Check sheet for the drawn part. Datum: minimum x, y, z corner. Units: mm. A direction names the side the tool comes from. Give positions to 0.01 mm unless a question says otherwise; leave off trailing zeros. Write each loop counter-clockwise with the first axis right and the second up, starting at its lowest first coordinate (ties: lowest second). Pieces come first, ordered by that corner, then holes.
(1) Depth check by flat-ended pin: P1, Ø2, axis at x = 19.5, z = 4, coming from the -Y side; P2, Ø4, axis at x = 82.5, z = 3.5, coming from the -Y side. Enter the tip coordinate at first touch or a pass-through.
(2) Thickness scan on line 1 along Y through (x, z) = (24, 2); line 2 along X through (y, z) = (23.5, 11.25); line 3 along Y through (x, z) = (28.5, 8). Record the ranges inside material, lowest first.
(3) Mould release check, pull along Y, two halves, no side actions. Record for the marked faces 4, 5, 6 and 7: +Y half, -Y half, draft (parallel to the pull), parting line (faces both ways), or undercut.
(4) Cross-section at C-C (y = 26.5). Record the boundary of the cut face in (x, z).
(5) Tool access check on the marked faces 1, 2 and 3. Record the directions out of +Z, -Z, +X, -X, +Y, -Y that give a thin tool (end or side, any length) a straight path to the whole face; none if there is none.
(6) Cross-section at B-B (x = 60.5). Record the boundary of the cut face in (y, z), and give its area (3 significant figures).
(7) Cross-section at A-A (y = 114). Record the boundary of the cut face in (x, z).
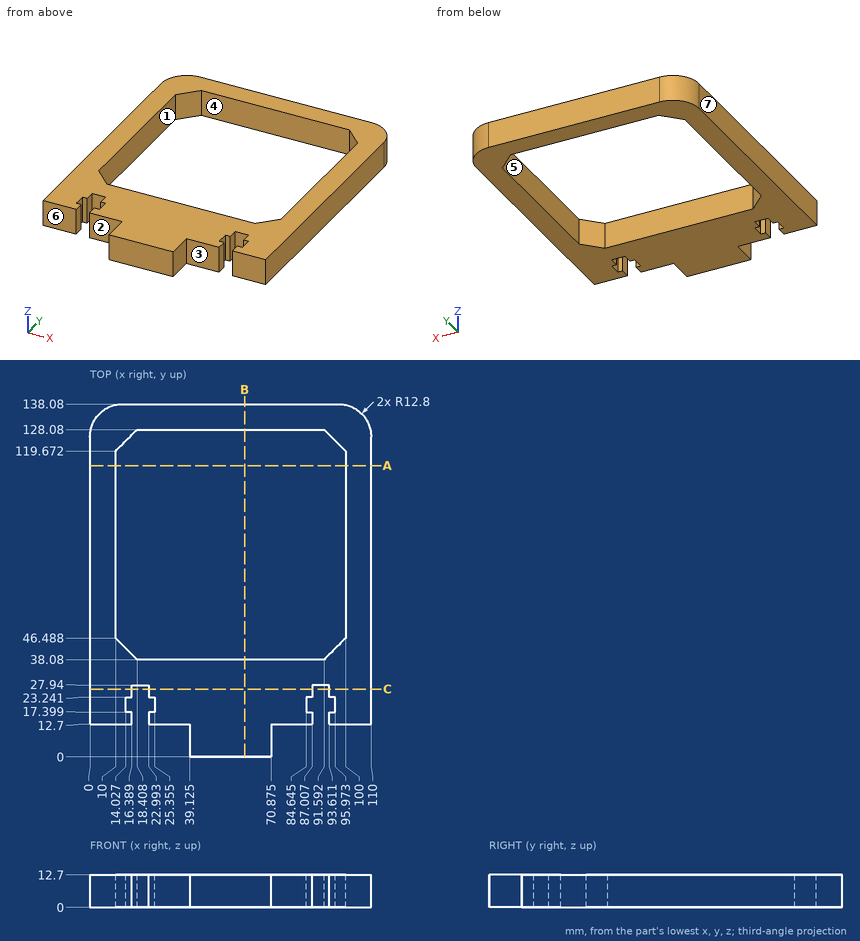
Reply:
1. P1: stops at y = 27.94
1. P2: stops at y = 12.7
2. line 1: y = 12.7 to 17.4, 23.24 to 38.08, 128.08 to 138.08
2. line 2: x = 0 to 16.39, 22.99 to 87.01, 93.61 to 110
2. line 3: y = 12.7 to 38.08, 128.08 to 138.08
3. face 4: undercut
3. face 5: undercut
3. face 6: -Y half
3. face 7: draft
4. outline: (0, 0) - (16.39, 0) - (16.39, 12.7) - (0, 12.7) - close; (22.99, 0) - (87.01, 0) - (87.01, 12.7) - (22.99, 12.7) - close; (93.61, 0) - (110, 0) - (110, 12.7) - (93.61, 12.7) - close
5. face 1: +Z, -Z
5. face 2: +Z, -Z, -X, -Y
5. face 3: +Z, -Z, +X, -Y
6. outline: (0, 0) - (38.08, 0) - (38.08, 12.7) - (0, 12.7) - close; (128.08, 0) - (138.08, 0) - (138.08, 12.7) - (128.08, 12.7) - close
6. area: 611 mm2
7. outline: (0, 0) - (10, 0) - (10, 12.7) - (0, 12.7) - close; (100, 0) - (110, 0) - (110, 12.7) - (100, 12.7) - close
